The listing builds one solid part. Answer for the finished solid, in the listing's coordinates (mm). Give positions to 0.01 mm unless a question says otherwise; leave off trailing zeros. Order: outer loops, then holes, each group sorted by start corner. A loop starts at its lowest first (then second) coordinate and runs counter-clockwise, first axis right, second up. Notation, with made-up numbers: (58, -21) - (86, -21) arc R27 cw to (86, 13) - close; hole circle Ø7 at (76, -2). An arc over 180 degrees is marked (long way). Use a Markdown table: item, result. Add a question column.
1) The mould has two halves that part along X. Classify faces 1 (the face through (2, 0, 2)), 2 (the face through (-49.14, 3.14, 45.54)): released by +X, released by -X, zero draft, split by the parting line, or undercut.
2) Find section A-A, the plane z = -45. Determine the outline of the cut face in (x, y) (3 decimals).
3) Straight lines are drawn through the part: line 1 (Z direction, x = -140, y = 1.75); line 2 (X direction, y = 1.75, z = -45) (3 decimals). For each, find the intervals that lie inside material, in ascending order.
4) Find section B-B, the plane x = -45. Determine the outline of the cut face in (y, z) (3 decimals), plus the area to 3 significant figures.
5) A flat-ended cylindrical pin translates along its axis: pin 1 (5 mm diameter, centred on x = -45, z = -45, fed in from -Y). Find the tip coordinate at first contact, or state that the pin passes through.
Autodesk Inventor part; units mm, degrees
ref_plane "YZ Plane" through (0, 0, 0) normal (1, 0, 0) x (0, 1, 0)
ref_plane "XZ Plane" through (0, 0, 0) normal (0, 1, 0) x (-1, 0, 0)
ref_plane "XY Plane" through (0, 0, 0) normal (0, 0, 1) x (1, 0, 0)
sketch "Sketch1" plane through (0, 0, 0) normal (0, 1, 0) x (-1, 0, 0)
  line L0 (150, -150) -> (-150, -150)
  line L1 (-150, -150) -> (-150, 150)
  line L2 (-150, 150) -> (150, 150)
  line L3 (150, 150) -> (150, -150)
  line L4 (150, -150) -> (-150, 150) construction
  line L5 (-150, -150) -> (150, 150) construction
  point P0 (0, 0)
  point P1 (45, 45)
  point P2 (-45, 45)
  point P3 (-45, -45)
  point P4 (45, -45)
  dimension "d0" = 300
  dimension "d1" = 300
  dimension "d2" = 45
  dimension "d4" = 45
  dimension "d5" = 45
  dimension "d6" = 45
extrude "Extrusion1" add sketch "Sketch1" along normal blind 6.2
hole "Hole1" at (-45, 0, 45) at (45, 0, 45) at (45, 0, -45) at (-45, 0, -45) direction (0, 1, 0) diameter 8.35 end through all
sketch "Sketch2" plane through (0, 6.2, 0) normal (0, 1, 0) x (1, 0, 0)
  line L0 (-150, -150) -> (150, -150)
  line L1 (-150, 150) -> (-150, -150)
  line L2 (150, 150) -> (-150, 150)
  line L3 (150, -150) -> (150, 150)
  point P0 (0, 0)
  point P1 (-140, -140)
  point P2 (140, -140)
  point P3 (140, 140)
  point P4 (-140, 140)
  dimension "d16" = 10
  dimension "d17" = 10
  dimension "d18" = 10
  dimension "d19" = 10
hole "Hole2" at (140, 6.2, 140) at (140, 6.2, -140) at (-140, 6.2, -140) at (-140, 6.2, 140) direction (0, -1, 0) diameter 4.5 end through all
properties part number "Base_Mdf" material "Wood (Birch)"
The answers:
| question | item | result |
|---|---|---|
| 1 | face 1 | zero draft |
| 1 | face 2 | undercut |
| 2 | outline | (-150, 0) - (-49.175, 0) - (-49.175, 6.2) - (-150, 6.2) - close; (-40.825, 0) - (40.825, 0) - (40.825, 6.2) - (-40.825, 6.2) - close; (49.175, 0) - (150, 0) - (150, 6.2) - (49.175, 6.2) - close |
| 3 | line 1 | -150 to -142.25, -137.75 to 137.75, 142.25 to 150 |
| 3 | line 2 | -150 to -49.175, -40.825 to 40.825, 49.175 to 150 |
| 4 | outline | (0, -150) - (6.2, -150) - (6.2, -49.175) - (0, -49.175) - close; (0, -40.825) - (6.2, -40.825) - (6.2, 40.825) - (0, 40.825) - close; (0, 49.175) - (6.2, 49.175) - (6.2, 150) - (0, 150) - close |
| 4 | area | 1,760 mm2 |
| 5 | pin 1 | through |
